from build123d import *

# Parameters (mm, degrees)
SKETCH6_W           = 115
SKETCH6_H           = 150
BOSS_EXTRUDE2_DEPTH = 4
SKETCH7_W           = 75
SKETCH7_H           = 15
CUT_EXTRUDE1_DEPTH  = 5
FILLET1_R           = 1
SKETCH8_W           = 10
SKETCH8_H           = 15
CUT_EXTRUDE2_DEPTH  = 5
FILLET2_R           = 1
CUT_EXTRUDE3_DEPTH  = 5
FILLET3_R           = 2
SKETCH14_R          = 1.5
CUT_EXTRUDE4_DEPTH  = 5
SKETCH17_R          = 1.5
CUT_EXTRUDE6_DEPTH  = 5
SKETCH18_R          = 1.5
CUT_EXTRUDE7_DEPTH  = 5


with BuildPart() as part:
    # Sketch6 → Boss-Extrude2 (new body)
    with BuildSketch(Plane.XY):
        with Locations((-57.5, 75)):
            Rectangle(SKETCH6_W, SKETCH6_H)
    extrude(amount=BOSS_EXTRUDE2_DEPTH)

    # Sketch7 → Cut-Extrude1 (cut, through all)
    with BuildSketch(Plane.XY.offset(4)):
        with Locations((-57.5, 7.5)):
            Rectangle(SKETCH7_W, SKETCH7_H)
    extrude(amount=-CUT_EXTRUDE1_DEPTH, mode=Mode.SUBTRACT)

    # Fillet1
    fillet1_edges = [part.edges().sort_by_distance(p)[0] for p in [
        (-95, 0, 2),
        (-95, 15, 2),
        (-20, 15, 2),
        (-20, 0, 2),
        (0, 0, 2),
        (-115, 0, 2),
    ]]
    fillet(fillet1_edges, radius=FILLET1_R)

    # Sketch8 → Cut-Extrude2 (cut, through all)
    with BuildSketch(Plane.XY.offset(4)):
        with Locations((-62.5, 142.5)):
            Rectangle(SKETCH8_W, SKETCH8_H)
        with Locations((-52.5, 142.5)):
            Rectangle(SKETCH8_W, SKETCH8_H)
    extrude(amount=-CUT_EXTRUDE2_DEPTH, mode=Mode.SUBTRACT)

    # Fillet2
    fillet2_edges = [part.edges().sort_by_distance(p)[0] for p in [
        (-67.5, 135, 2),
        (-67.5, 150, 2),
        (-47.5, 150, 2),
        (-47.5, 135, 2),
    ]]
    fillet(fillet2_edges, radius=FILLET2_R)

    # Sketch11 → Cut-Extrude3 (cut, through all)
    with BuildSketch(Plane.XY.offset(4)):
        Polygon((-87.5, 150), (-115, 50), (-115, 150), align=None)
        Polygon((0, 50), (0, 150), (-27.5, 150), align=None)
    extrude(amount=-CUT_EXTRUDE3_DEPTH, mode=Mode.SUBTRACT)

    # Fillet3
    fillet3_edges = [part.edges().sort_by_distance(p)[0] for p in [
        (0, 50, 2),
        (-27.5, 150, 2),
        (-87.5, 150, 2),
        (-115, 50, 2),
    ]]
    fillet(fillet3_edges, radius=FILLET3_R)

    # Sketch14 → Cut-Extrude4 (cut, through all)
    with BuildSketch(Plane(origin=(0, 0, 0), x_dir=(-1, 0, 0), z_dir=(0, 0, -1))):
        with Locations((40, 144)):
            Circle(SKETCH14_R)
        with Locations((75, 144)):
            Circle(SKETCH14_R)
    extrude(amount=-CUT_EXTRUDE4_DEPTH, mode=Mode.SUBTRACT)

    # Sketch17 → Cut-Extrude6 (cut, through all)
    with BuildSketch(Plane.XY.offset(4)):
        with Locations((-76.19, 121.74)):
            Circle(SKETCH17_R)
        with Locations((-38.81, 121.74)):
            Circle(SKETCH17_R)
        with Locations((-76.19, 85)):
            Circle(SKETCH17_R)
        with Locations((-38.81, 85)):
            Circle(SKETCH17_R)
    extrude(amount=-CUT_EXTRUDE6_DEPTH, mode=Mode.SUBTRACT)

    # Sketch18 → Cut-Extrude7 (cut, through all)
    with BuildSketch(Plane.XY.offset(4)):
        with Locations((-84, 18)):
            Circle(SKETCH18_R)
        with Locations((-40.9, 68.8)):
            Circle(SKETCH18_R)
    extrude(amount=-CUT_EXTRUDE7_DEPTH, mode=Mode.SUBTRACT)


solid = part.part
Part model, mm, in its own coordinate system. A direction names the side the tool comes from. Give positions to 0.01 mm unless a question says otherwise; leave off trailing zeros. Loops run counter-clockwise (first coordinate to the right, second up) from the corner with the lowest first, then second, coordinate; pieces in that order, holes last.
(1) Band-saw the part on D-D (x = -16). Write the cut outline in (y, z).
Return value:
outline: (0, 0) - (108.18, 0) - (108.18, 4) - (0, 4) - close
(2) Drill centre lines: line 1 along X through (y, z) = (122, 3.55); line 2 along X through (y, z) = (123, 1.2) (3 decimals); line 3 along Y through (x, z) = (-38.81, 2.35). Where is each one in solid material? Low to high.
Return value:
line 1: x = -95.2 to -77.67, -74.71 to -40.29, -37.33 to -19.8
line 2: x = -94.925 to -77.004, -75.376 to -39.624, -37.996 to -20.075
line 3: y = 15 to 83.5, 86.5 to 120.24, 123.24 to 143.09, 144.91 to 150
(3) 3-axis set-ups, long thin cutter, end or side, ignore diameter. For faces 1 (the cylindrical face through (-41.225, 67.336, 2.028)), 2 (the flat face through (-20, 7, 2)), 3 (the flat face through (-47.5, 142, 2)): which of +Z, -Z, +X, -X, +Y, -Y reach the whole face in a straight line?
Return value:
face 1: +Z, -Z
face 2: +Z, -Z, -Y
face 3: +Z, -Z, +Y
(4) Pin check, flat tips, straight feed: pin 1 (2 mm diameter, centred on x = -72.5, z = 2.5, fed in from -Y); pin 2 (2 mm diameter, centred on x = -60, z = 3, fed in from +Y); pin 3 (1.2 mm diameter, centred on y = 140.5, z = 2.5, fed in from -X). Stop position of each tip, or through.
Return value:
pin 1: stops at y = 15
pin 2: stops at y = 135
pin 3: stops at x = -90.28
(5) Band-saw the part on A-A (y = 138.5). Write the cut outline in (x, z), and give its area (3 significant figures).
Return value:
outline: (-90.66, 0) - (-67.5, 0) - (-67.5, 4) - (-90.66, 4) - close; (-47.5, 0) - (-24.34, 0) - (-24.34, 4) - (-47.5, 4) - close
area: 185 mm2
(6) Pull direction X, two halves, no side cores. Call faces 4 (the flat face through (-77, 150, 2)), 5 (the flat face through (-115, 25, 2)), 6 (the cylindrical face through (-39.805, 145.487, 1.972)): pulls with the +X half, pulls with the -X half, needs draft (parallel to the pull), parting line crosses it, or undercut.
Return value:
face 4: needs draft
face 5: pulls with the -X half
face 6: undercut
(7) Band-saw the part on C-C (y = 73). Write the cut outline in (x, z) (3 decimals).
Return value:
outline: (-108.675, 0) - (-6.325, 0) - (-6.325, 4) - (-108.675, 4) - close
(8) Band-saw the part on B-B (z = 3.4). Count the separate pieces of the cut face and the enclosed holes in it, and give its area (3 significant figures).
Return value:
separate pieces: 1
enclosed holes: 8
area: 13,000 mm2
